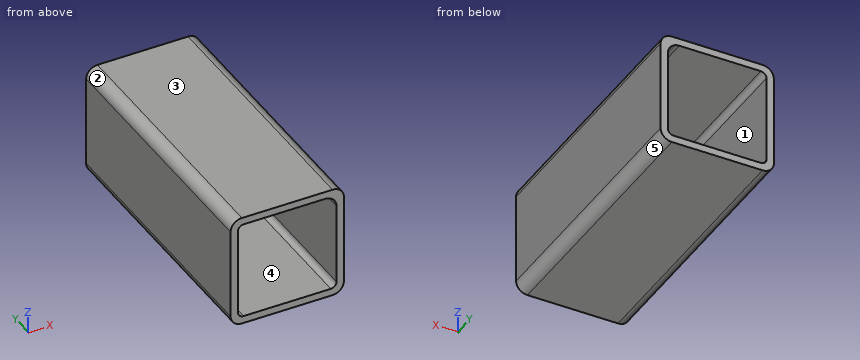
```python
from build123d import *

# Parameters (mm, degrees)
F0_W     = 40
F0_H     = 40
F0_W_2   = 34.8
F0_H_2   = 34.8
F1_DEPTH = 94
F2_R     = 4
F3_R     = 2


with BuildPart() as f1:
    # F0 (on Front) → F1 (new body)
    with BuildSketch(Plane.XZ):
        Rectangle(F0_W, F0_H)
        Rectangle(F0_W_2, F0_H_2, mode=Mode.SUBTRACT)
    extrude(amount=F1_DEPTH)

    # F2
    f2_edges = [f1.edges().sort_by_distance(p)[0] for p in [
        (20, -47, 20),
        (-20, -47, 20),
        (20, -47, -20),
        (-20, -47, -20),
        (17.4, -47, 17.4),
    ]]
    fillet(f2_edges, radius=F2_R)

    # F3
    f3_edges = [f1.edges().sort_by_distance(p)[0] for p in [
        (-17.4, -47, 17.4),
        (-17.4, -47, -17.4),
        (17.4, -47, -17.4),
        (16, -47, 20),
    ]]
    fillet(f3_edges, radius=F3_R)


solid = f1.part
```
Here's how the part is built. I have some questions about the finished solid (model axes, mm). Face numbers are marked on the shaded views. A direction names the side the tool comes from. Round coordinates to 2 decimals unless told otherwise and drop trailing zeros. Write each loop counter-clockwise with the first axis right and the second up, starting at its lowest first coordinate (ties: lowest second). Pieces come first, ordered by that corner, then holes. Notation, with made-up numbers: M -5,40 L 52,40 A36 ccw 52,74 Z; hole C 22.5,49.25 d2. An arc over 180 degrees is marked long. Answer as CSV lines item,"result". Start each with the question number.
1. Suppose I cut it at B-B on z = -2.5. Write out the boundary of the cut face in (x, y).
2. I need wall thicknesses on probe 1 along X at (y, z) = (-21.5, 12); probe 2 along Z at (x, y) = (-16, -9). Which ranges of each line are inside material? Lowest first, please.
3. Suppose I cut it at C-C on y = -74.5. Write out the boundary of the cut face in (x, z).
4. On a 3-axis mill with a long thin cutter (end or side, diameter ignored), from which of +Z, -Z, +X, -X, +Y, -Y can I reach the whole of each face in a straight line? I mean the marked faces 1 and 2. Say none if no direction works.
5. Suppose I cut it at A-A on x = -8. Write out the boundary of the cut face in (y, z).
6. Thinking about a two-plate mould opening in X: for the marked faces 3, 4 and 5, which applies, released by +X, released by -X, zero draft, split by the parting line, or undercut?
Check result:
1,outline,"M -20,-94 L -17.4,-94 L -17.4,0 L -20,0 Z; M 17.4,-94 L 20,-94 L 20,0 L 17.4,0 Z"
2,probe 1,"x = -20 to -17.4, 17.4 to 20"
2,probe 2,"z = -20 to -17.31, 17.31 to 20"
3,outline,"M -20,-16 A4 ccw -16,-20 L 16,-20 A4 ccw 20,-16 L 20,16 A4 ccw 16,20 L -16,20 A4 ccw -20,16 Z; hole M -17.4,-15.4 A2 ccw -15.4,-17.4 L 15.4,-17.4 A2 ccw 17.4,-15.4 L 17.4,13.4 A4 ccw 13.4,17.4 L -15.4,17.4 A2 ccw -17.4,15.4 Z"
4,face 1,"+Y, -Y"
4,face 2,"+Z, -X, +Y, -Y"
5,outline,"M -94,-20 L 0,-20 L 0,-17.4 L -94,-17.4 Z; M -94,17.4 L 0,17.4 L 0,20 L -94,20 Z"
6,face 3,"zero draft"
6,face 4,"undercut"
6,face 5,"released by +X"
